Autodesk Inventor part; units mm, degrees
ref_plane "YZ Plane" through (0, 0, 0) normal (1, 0, 0) x (0, 1, 0)
ref_plane "XZ Plane" through (0, 0, 0) normal (0, 1, 0) x (-1, 0, 0)
ref_plane "XY Plane" through (0, 0, 0) normal (0, 0, 1) x (1, 0, 0)
sketch "Boceto1" plane through (0, 0, 0) normal (1, 0, 0) x (0, 1, 0)
  line L0 (0, 45.315) -> (20, 45.315)
  line L1 (35, 30.315) -> (35, -29.685)
  line L2 (20, -44.685) -> (0, -44.685)
  arc A0 (35, 30.315) -> (20, 45.315) centre (20, 30.315) ccw
  arc A1 (20, -44.685) -> (35, -29.685) centre (20, -29.685) ccw
  point P0 (0, 0)
  point P1 (35, 45.315)
  point P2 (35, -44.685)
  dimension "d0" = 35
  dimension "d1" = 90
  dimension "d2" = 15
sketch "Boceto2" plane through (0, 0, 0) normal (0, 1, 0) x (-1, 0, 0)
  circle A0 centre (0, 45) radius 3
  point P0 (0, 0)
  dimension "d3" = 6
sweep "Barrido1" add profiles "Boceto2" path "Boceto1"
properties part number "AGARRADERA" material "Acero inoxidable"
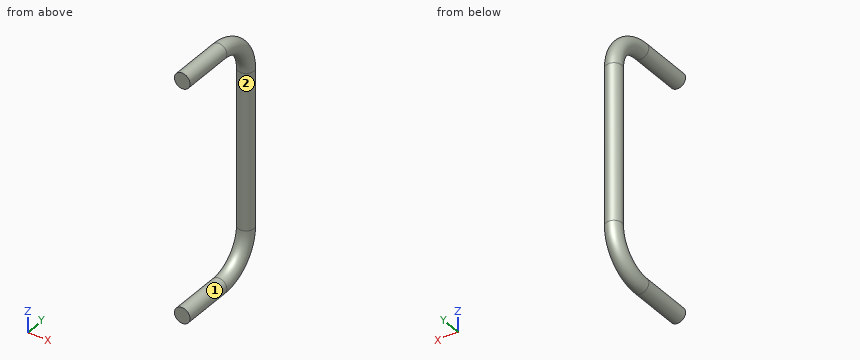
Model file for the job. Use its own axes, mm. Face numbers are marked on the shaded views. A direction names the side the tool comes from. Coordinates: 2 decimals unless noted, no trailing zeros. Write each loop counter-clockwise with the first axis right and the second up, starting at its lowest first coordinate (ties: lowest second). Pieces come first, ordered by that corner, then holes. Notation, with made-up numbers: (-17, -10) - (-10, -10) arc R11 ccw to (-10, -5) - close; hole circle Ø1 at (-20.5, 2). An arc over 180 degrees is marked (long way). Use a Markdown table: item, result. Add a question column.
Item 1: Drill centre lines: line 1 along Z through (x, y) = (-0.25, 11.5); line 2 along Z through (x, y) = (2.25, 18); line 3 along Y through (x, z) = (0.25, 2). Where is each one in solid material? Low to high.
Item 2: Band-saw the part on B-B, the plane y = 15.5. Write the cut outline in (x, z), and give its area (3 significant figures).
Item 3: 3-axis set-ups, long thin cutter, end or side, ignore diameter. For the marked faces 1 and 2: which of +Z, -Z, +X, -X, +Y, -Y reach the whole face in a straight line?
Item 4: Band-saw the part on A-A, the plane x = 0. Write the cut outline in (y, z) (3 decimals), and give its area (3 significant figures).
Item 5: Drop flat-ended pins along their axis: pin 1 (2 mm diameter, centred on x = 0.5, y = 24, fed in from -Z); pin 2 (3 mm diameter, centred on x = -1.5, y = 33.5, fed in from -Z); pin 3 (1 mm diameter, centred on y = 32.5, z = -22.5, fed in from +X). Give the stop position or say it passes through.
Item 6: Band-saw the part on C-C, the plane z = -1. Write the cut outline in (x, y) (3 decimals), and give its area (3 significant figures).
A:
| question | item | result |
|---|---|---|
| 1 | line 1 | z = -47.36 to -41.38, 42.01 to 47.99 |
| 1 | line 2 | z = -46.35 to -42.39, 43.02 to 46.98 |
| 1 | line 3 | y = 31.7 to 37.67 |
| 2 | outline | circle Ø6 at (0, -44.37); circle Ø6 at (0, 45) |
| 2 | area | 56.5 mm² |
| 3 | face 1 | -Y |
| 3 | face 2 | none |
| 4 | outline | (0, -47.37) - (20, -47.37) arc R17.685 ccw to (37.685, -29.685) - (37.685, 30.315) arc R17.685 ccw to (20, 48) - (0, 48) - (0, 42) - (20, 42) arc R11.685 cw to (31.685, 30.315) - (31.685, -29.685) arc R11.685 cw to (20, -41.37) - (0, -41.37) - close |
| 4 | area | 877 mm² |
| 5 | pin 1 | stops at z = -47.1 |
| 5 | pin 2 | stops at z = -42.37 |
| 5 | pin 3 | stops at x = 2.48 |
| 6 | outline | circle Ø6 at (0, 34.685) |
| 6 | area | 28.3 mm² |
